Geometry check sheet. Reference: the model listing, model coordinates, mm. Round coordinates to 2 decimals unless told otherwise and drop trailing zeros. Order: outer loops, then holes, each group sorted by start corner. A loop starts at its lowest first (then second) coordinate and runs counter-clockwise, first axis right, second up. Notation, with made-up numbers: (-34, 14.25) - (-10, 14.25) arc R28 cw to (-10, 43.25) - close; hole circle Ø4 at (12, 12.25). An arc over 180 degrees is marked (long way). Return JSON: item names as keys, results as strings. Group by question number.
Q1. Sectioned sample at B-B, the plane z = 26. Record the cut outline in (x, y), then the cut area to 3 significant figures.
Q2. Gauge pin test, flat ends, axial feed: pin 1 Ø1.4 at (x, z) = (2, -30) entering from +Y; pin 2 Ø3 at (x, y) = (2.5, -126) entering from +Z; pin 3 Ø1.5 at (x, y) = (1, -33) entering from -Z. Record the tip position at first contact, or that the pin passes through.
Q3. Sectioned sample at A-A, the plane y = -115. Record the cut outline in (x, z), then the cut area to 3 significant figures.
Q4. Material ranges on line 1 along Z through (x, y) = (4.5, 34); line 2 along Y through (x, z) = (3, -27); line 3 along Y through (x, z) = (2.5, -20), recorded low to high.
```python
from build123d import *

# Parameters (mm, degrees)
F1_DEPTH = 6.35


with BuildPart() as f1:
    # F0 (on Right) → F1 (new body)
    with BuildSketch(Plane.YZ):
        with BuildLine():
            Line((-77.7875, 34.144226), (-100.0125, 34.144226))
            ThreePointArc((-100.0125, 34.144226), (-101.6, 32.556726), (-103.1875, 34.144226))
            Line((-103.1875, 34.144226), (-139.7, 34.144226))
            Line((-139.7, 34.144226), (-139.7, -26.180774))
            Line((-139.7, -26.180774), (-103.1875, -26.180774))
            ThreePointArc((-103.1875, -26.180774), (-101.6, -24.593274), (-100.0125, -26.180774))
            Line((-100.0125, -26.180774), (-77.7875, -26.180774))
            ThreePointArc((-77.7875, -26.180774), (-76.2, -24.593274), (-74.6125, -26.180774))
            Line((-74.6125, -26.180774), (-26.9875, -26.180774))
            ThreePointArc((-26.9875, -26.180774), (-25.4, -24.593274), (-23.8125, -26.180774))
            Line((-23.8125, -26.180774), (-1.5875, -26.180774))
            ThreePointArc((-1.5875, -26.180774), (0, -24.593274), (1.5875, -26.180774))
            Line((1.5875, -26.180774), (49.2125, -26.180774))
            ThreePointArc((49.2125, -26.180774), (50.8, -24.593274), (52.3875, -26.180774))
            Line((52.3875, -26.180774), (74.6125, -26.180774))
            ThreePointArc((74.6125, -26.180774), (76.2, -24.593274), (77.7875, -26.180774))
            Line((77.7875, -26.180774), (125.4125, -26.180774))
            ThreePointArc((125.4125, -26.180774), (127, -24.593274), (128.5875, -26.180774))
            Line((128.5875, -26.180774), (150.8125, -26.180774))
            ThreePointArc((150.8125, -26.180774), (152.4, -24.593274), (153.9875, -26.180774))
            Line((153.9875, -26.180774), (171.45, -26.180774))
            Line((171.45, -26.180774), (171.45, -13.480774))
            ThreePointArc((171.45, -13.480774), (169.8625, -11.893274), (171.45, -10.305774))
            Line((171.45, -10.305774), (171.45, 18.269226))
            ThreePointArc((171.45, 18.269226), (169.8625, 19.856726), (171.45, 21.444226))
            Line((171.45, 21.444226), (171.45, 34.144226))
            Line((171.45, 34.144226), (153.9875, 34.144226))
            ThreePointArc((153.9875, 34.144226), (152.4, 32.556726), (150.8125, 34.144226))
            Line((150.8125, 34.144226), (128.5875, 34.144226))
            ThreePointArc((128.5875, 34.144226), (127, 32.556726), (125.4125, 34.144226))
            Line((125.4125, 34.144226), (77.7875, 34.144226))
            ThreePointArc((77.7875, 34.144226), (76.2, 32.556726), (74.6125, 34.144226))
            Line((74.6125, 34.144226), (52.3875, 34.144226))
            ThreePointArc((52.3875, 34.144226), (50.8, 32.556726), (49.2125, 34.144226))
            Line((49.2125, 34.144226), (1.5875, 34.144226))
            ThreePointArc((1.5875, 34.144226), (0, 32.556726), (-1.5875, 34.144226))
            Line((-1.5875, 34.144226), (-23.8125, 34.144226))
            ThreePointArc((-23.8125, 34.144226), (-25.4, 32.556726), (-26.9875, 34.144226))
            Line((-26.9875, 34.144226), (-74.6125, 34.144226))
            ThreePointArc((-74.6125, 34.144226), (-76.2, 32.556726), (-77.7875, 34.144226))
        make_face()
        with BuildLine():
            ThreePointArc((-101.6, 35.731726), (-100.477468, 35.266758), (-100.0125, 34.144226))
            Line((-100.0125, 34.144226), (-77.7875, 34.144226))
            ThreePointArc((-77.7875, 34.144226), (-77.322532, 35.266758), (-76.2, 35.731726))
            Line((-76.2, 35.731726), (-76.2, 40.494226))
            Line((-76.2, 40.494226), (-101.6, 40.494226))
            Line((-101.6, 40.494226), (-101.6, 35.731726))
        make_face()
        with BuildLine():
            Line((-25.4, 40.494226), (-25.4, 35.731726))
            ThreePointArc((-25.4, 35.731726), (-24.277468, 35.266758), (-23.8125, 34.144226))
            Line((-23.8125, 34.144226), (-1.5875, 34.144226))
            ThreePointArc((-1.5875, 34.144226), (-1.122532, 35.266758), (0, 35.731726))
            Line((0, 35.731726), (0, 40.494226))
            Line((0, 40.494226), (-25.4, 40.494226))
        make_face()
        with BuildLine():
            Line((50.8, 40.494226), (50.8, 35.731726))
            ThreePointArc((50.8, 35.731726), (51.922532, 35.266758), (52.3875, 34.144226))
            Line((52.3875, 34.144226), (74.6125, 34.144226))
            ThreePointArc((74.6125, 34.144226), (75.077468, 35.266758), (76.2, 35.731726))
            Line((76.2, 35.731726), (76.2, 40.494226))
            Line((76.2, 40.494226), (50.8, 40.494226))
        make_face()
        with BuildLine():
            Line((127, 40.494226), (127, 35.731726))
            ThreePointArc((127, 35.731726), (128.122532, 35.266758), (128.5875, 34.144226))
            Line((128.5875, 34.144226), (150.8125, 34.144226))
            ThreePointArc((150.8125, 34.144226), (151.277468, 35.266758), (152.4, 35.731726))
            Line((152.4, 35.731726), (152.4, 40.494226))
            Line((152.4, 40.494226), (127, 40.494226))
        make_face()
        with BuildLine():
            Line((177.8, 19.856726), (173.0375, 19.856726))
            ThreePointArc((173.0375, 19.856726), (172.572532, 18.734194), (171.45, 18.269226))
            Line((171.45, 18.269226), (171.45, -10.305774))
            ThreePointArc((171.45, -10.305774), (172.572532, -10.770742), (173.0375, -11.893274))
            Line((173.0375, -11.893274), (177.8, -11.893274))
            Line((177.8, -11.893274), (177.8, 19.856726))
        make_face()
        with BuildLine():
            Line((150.8125, -26.180774), (128.5875, -26.180774))
            ThreePointArc((128.5875, -26.180774), (128.122532, -27.303306), (127, -27.768274))
            Line((127, -27.768274), (127, -32.530774))
            Line((127, -32.530774), (152.4, -32.530774))
            Line((152.4, -32.530774), (152.4, -27.768274))
            ThreePointArc((152.4, -27.768274), (151.277468, -27.303306), (150.8125, -26.180774))
        make_face()
        with BuildLine():
            Line((74.6125, -26.180774), (52.3875, -26.180774))
            ThreePointArc((52.3875, -26.180774), (51.922532, -27.303306), (50.8, -27.768274))
            Line((50.8, -27.768274), (50.8, -32.530774))
            Line((50.8, -32.530774), (76.2, -32.530774))
            Line((76.2, -32.530774), (76.2, -27.768274))
            ThreePointArc((76.2, -27.768274), (75.077468, -27.303306), (74.6125, -26.180774))
        make_face()
        with BuildLine():
            Line((-1.5875, -26.180774), (-23.8125, -26.180774))
            ThreePointArc((-23.8125, -26.180774), (-24.277468, -27.303306), (-25.4, -27.768274))
            Line((-25.4, -27.768274), (-25.4, -32.530774))
            Line((-25.4, -32.530774), (0, -32.530774))
            Line((0, -32.530774), (0, -27.768274))
            ThreePointArc((0, -27.768274), (-1.122532, -27.303306), (-1.5875, -26.180774))
        make_face()
        with BuildLine():
            Line((-77.7875, -26.180774), (-100.0125, -26.180774))
            ThreePointArc((-100.0125, -26.180774), (-100.477468, -27.303306), (-101.6, -27.768274))
            Line((-101.6, -27.768274), (-101.6, -32.530774))
            Line((-101.6, -32.530774), (-76.2, -32.530774))
            Line((-76.2, -32.530774), (-76.2, -27.768274))
            ThreePointArc((-76.2, -27.768274), (-77.322532, -27.303306), (-77.7875, -26.180774))
        make_face()
    extrude(amount=F1_DEPTH)


solid = f1.part
```
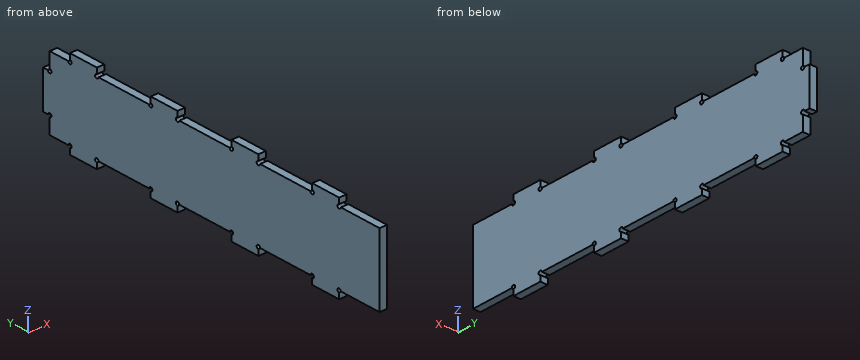
Reply:
{
 "1": {"outline": "(0, -139.7) - (6.35, -139.7) - (6.35, 171.45) - (0, 171.45) - close", "area": "1,980 mm^2"},
 "2": {"pin 1": "y = 152.4", "pin 2": "z = 34.14", "pin 3": "z = -26.18"},
 "3": {"outline": "(0, -26.18) - (6.35, -26.18) - (6.35, 34.14) - (0, 34.14) - close", "area": "383 mm^2"},
 "4": {"line 1": "-26.18 to 34.14", "line 2": "-100.24 to -77.56, -24.04 to -1.36, 52.16 to 74.84, 128.36 to 151.04", "line 3": "-139.7 to 171.45"}
}
